Work out the finished part from the listing and answer in its coordinate system (mm). A direction names the side the tool comes from. Give positions to 0.01 mm unless a question says otherwise; leave off trailing zeros. Loops run counter-clockwise (first coordinate to the right, second up) from the corner with the lowest first, then second, coordinate; pieces in that order, holes last.
from build123d import *

# Parameters (mm, degrees)
BOSS_EXTRUDE1_DEPTH = 37.6
CUT_EXTRUDE1_DEPTH  = 69.310699879
SKETCH4_R           = 1.6
CUT_EXTRUDE2_DEPTH  = 81.972748235
SKETCH5_R           = 1.65
CUT_EXTRUDE4_DEPTH  = 69.310699879
CUT_EXTRUDE5_DEPTH  = 69.310699879


with BuildPart() as part:
    # Sketch1 → Boss-Extrude1 (new body)
    with BuildSketch(Plane(origin=(0, 0, 0), x_dir=(0, 0, -1), z_dir=(1, 0, 0))):
        with BuildLine():
            Line((-9.866078609, -8.756426748), (-59.066078609, -8.756426748))
            Line((-59.066078609, -8.756426748), (-59.066078609, 28.843573252))
            Line((-59.066078609, 28.843573252), (-61.066078609, 28.843573252))
            Line((-61.066078609, 28.843573252), (-61.066078609, -9.756426748))
            ThreePointArc((-61.066078609, -9.756426748), (-60.77318539, -10.463533529), (-60.066078609, -10.756426748))
            Line((-60.066078609, -10.756426748), (-9.866078609, -10.756426748))
            Line((-9.866078609, -10.756426748), (-9.866078609, -8.756426748))
        make_face()
    extrude(amount=BOSS_EXTRUDE1_DEPTH)

    # Sketch3 → Cut-Extrude1 (cut, through all)
    with BuildSketch(Plane(origin=(0, 0, 59.066078609), x_dir=(-1, 0, 0), z_dir=(0, 0, -1))):
        with BuildLine():
            Line((-12.2, 17.689945041), (-12.2, 3.689945041))
            ThreePointArc((-12.2, 3.689945041), (-18.8, -2.910054959), (-25.4, 3.689945041))
            Line((-25.4, 3.689945041), (-25.4, 17.689945041))
            ThreePointArc((-25.4, 17.689945041), (-18.8, 24.289945041), (-12.2, 17.689945041))
        make_face()
    extrude(amount=-CUT_EXTRUDE1_DEPTH, mode=Mode.SUBTRACT)

    # Sketch4 → Cut-Extrude2 (cut, through all)
    with BuildSketch(Plane(origin=(0, -8.756426748, 0), x_dir=(1, 0, 0), z_dir=(0, 1, 0))):
        with Locations(Location((3.2, -14.566078609, 0), (0, 0, 270))):
            Circle(SKETCH4_R)
        with Locations(Location((3.2, -27.366078609, 0), (0, 0, 270))):
            Circle(SKETCH4_R)
        with Locations(Location((3.2, -20.966078609, 0), (0, 0, 270))):
            Circle(SKETCH4_R)
        with Locations(Location((3.2, -33.766078609, 0), (0, 0, 270))):
            Circle(SKETCH4_R)
        with Locations(Location((3.2, -40.166078609, 0), (0, 0, 270))):
            Circle(SKETCH4_R)
        with Locations(Location((3.2, -46.566078609, 0), (0, 0, 270))):
            Circle(SKETCH4_R)
        with Locations(Location((3.2, -52.966078609, 0), (0, 0, 270))):
            Circle(SKETCH4_R)
        with Locations(Location((34.4, -52.966078609, 0), (0, 0, 270))):
            Circle(SKETCH4_R)
        with Locations(Location((34.4, -46.566078609, 0), (0, 0, 270))):
            Circle(SKETCH4_R)
        with Locations(Location((34.4, -40.166078609, 0), (0, 0, 270))):
            Circle(SKETCH4_R)
        with Locations(Location((34.4, -27.366078609, 0), (0, 0, 270))):
            Circle(SKETCH4_R)
        with Locations(Location((34.4, -20.966078609, 0), (0, 0, 270))):
            Circle(SKETCH4_R)
        with Locations(Location((34.4, -33.766078609, 0), (0, 0, 270))):
            Circle(SKETCH4_R)
        with Locations(Location((34.4, -14.566078609, 0), (0, 0, 270))):
            Circle(SKETCH4_R)
    extrude(amount=-CUT_EXTRUDE2_DEPTH, mode=Mode.SUBTRACT)

    # Sketch5 → Cut-Extrude4 (cut, through all)
    with BuildSketch(Plane(origin=(0, 0, 59.066078609), x_dir=(-1, 0, 0), z_dir=(0, 0, -1))):
        with Locations((-26.55, 24.1133388)):
            Circle(SKETCH5_R)
        with Locations((-11.05, 24.1133388)):
            Circle(SKETCH5_R)
        with Locations((-3.3, 10.689945041)):
            Circle(SKETCH5_R)
        with Locations((-11.05, -2.733448718)):
            Circle(SKETCH5_R)
        with Locations((-34.3, 10.689945041)):
            Circle(SKETCH5_R)
        with Locations((-26.55, -2.733448718)):
            Circle(SKETCH5_R)
    extrude(amount=-CUT_EXTRUDE4_DEPTH, mode=Mode.SUBTRACT)

    # Sketch6 → Cut-Extrude5 (cut, through all)
    with BuildSketch(Plane(origin=(0, 0, 59.066078609), x_dir=(-1, 0, 0), z_dir=(0, 0, -1))):
        with BuildLine():
            Line((-37.6, 28.843573252), (-37.6, 10.043573252))
            ThreePointArc((-37.6, 10.043573252), (-32.093607486, 23.337180738), (-18.8, 28.843573252))
            Line((-18.8, 28.843573252), (-37.6, 28.843573252))
        make_face()
        with BuildLine():
            Line((0, 28.843573252), (-18.8, 28.843573252))
            ThreePointArc((-18.8, 28.843573252), (-5.506392514, 23.337180738), (0, 10.043573252))
            Line((0, 10.043573252), (0, 28.843573252))
        make_face()
    extrude(amount=-CUT_EXTRUDE5_DEPTH, mode=Mode.SUBTRACT)


solid = part.part
Item 1: Find section C-C, the plane y = 25. Write down the section's boundary in (x, z).
Item 2: Determine the mould class of faces 3 (the face through (37.6, -9, 41)), 4 (the face through (19, -10, 9.866)), 5 (the face through (32.838, -9.742, 46.219)) for opening direction X: released by +X, released by -X, zero draft, split by the parting line, or undercut.
Item 3: Find section D-D, the plane x = 18. Write down the section's boundary in (y, z).
Item 4: For faces 1 (the face through (3.27, -9.742, 25.768)), 2 (the face through (12.2, 11, 60)), determine the directions among +Z, -Z, +X, -X, +Y, -Y from which every point of the face is accessible in a straight line to the end or side of a thin tool.
Item 5: Consider line 1 (Y direction, x = 12.5, z = 20); line 2 (Z direction, x = 6.5, y = 12); line 3 (Y direction, x = 26, z = 60). Determine where each line is inside the solid, lowest interval first.
Item 6: Find section A-A, the plane y = 6. Write down the section's boundary in (x, z).
Item 7: Flat-ended cylindrical pins translate along their axes: pin 1 Ø1.5 at (x, z) = (32, 30.5) entering from +Y; pin 2 Ø2 at (x, y) = (3.3, 10.69) entering from -Z; pin 3 Ø4 at (x, y) = (10.5, 13) entering from -Z. Find the tip coordinate at first contact, or state that the pin passes through.
Item 8: Find section B-B, the plane x = 26.55. Write down the section's boundary in (y, z), plus the area to 3 significant figures.
Ans:
1. outline: (7.41, 59.07) - (9.66, 59.07) - (9.66, 61.07) - (7.41, 61.07) - close; (12.44, 59.07) - (25.16, 59.07) - (25.16, 61.07) - (12.44, 61.07) - close; (27.94, 59.07) - (30.19, 59.07) - (30.19, 61.07) - (27.94, 61.07) - close
2. face 3: released by +X
2. face 4: zero draft
2. face 5: undercut
3. outline: (-10.76, 9.87) - (-8.76, 9.87) - (-8.76, 59.07) - (-2.86, 59.07) - (-2.86, 61.07) - (-9.76, 61.07) arc R1 ccw to (-10.76, 60.07) - close; (24.24, 59.07) - (28.83, 59.07) - (28.83, 61.07) - (24.24, 61.07) - close
4. face 1: +Y, -Y
4. face 2: +Z, -Z
5. line 1: y = -10.76 to -8.76
5. line 2: z = 59.07 to 61.07
5. line 3: y = -10.76 to -4.29, -1.18 to 22.56, 25.67 to 27.41
6. outline: (0, 59.07) - (12.2, 59.07) - (12.2, 61.07) - (0, 61.07) - close; (25.4, 59.07) - (37.6, 59.07) - (37.6, 61.07) - (25.4, 61.07) - close
7. pin 1: stops at y = -8.76
7. pin 2: passes through
7. pin 3: stops at z = 59.07
8. outline: (-10.76, 9.87) - (-8.76, 9.87) - (-8.76, 59.07) - (-4.38, 59.07) - (-4.38, 61.07) - (-9.76, 61.07) arc R1 ccw to (-10.76, 60.07) - close; (-1.08, 59.07) - (22.46, 59.07) - (22.46, 61.07) - (-1.08, 61.07) - close; (25.76, 59.07) - (27.17, 59.07) - (27.17, 61.07) - (25.76, 61.07) - close
8. area: 161 mm2
